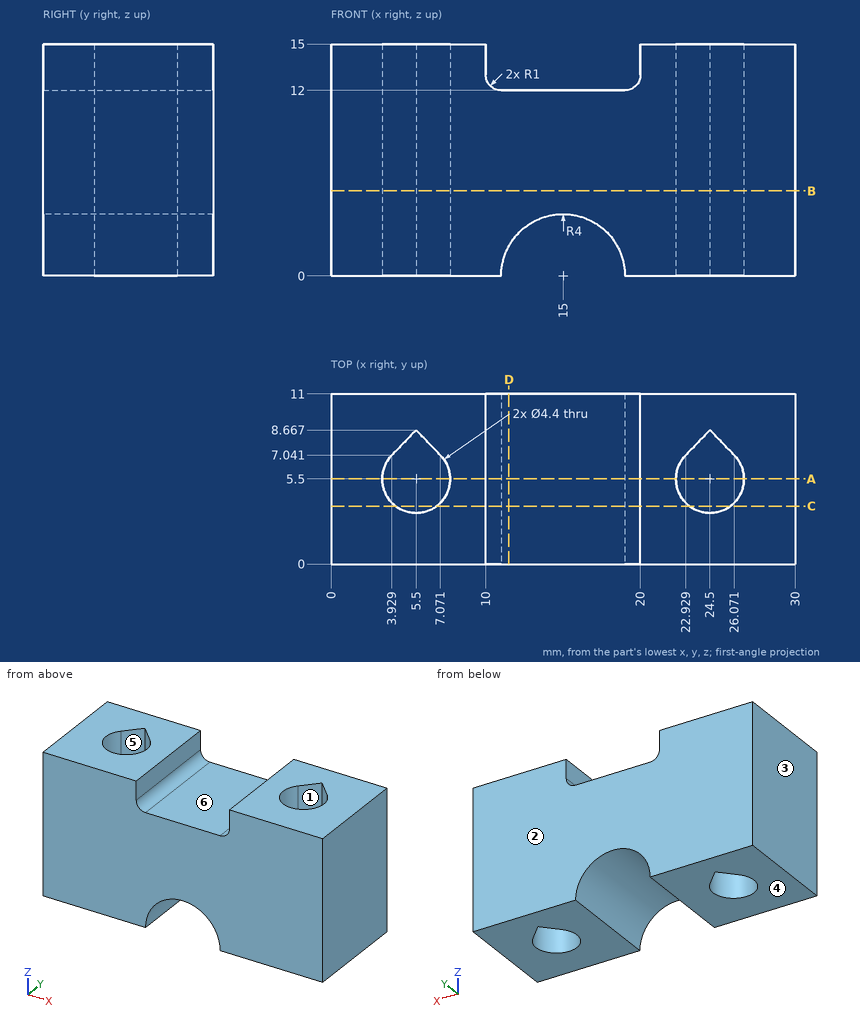
Study the drawing (mm; zero at the part's minimum x, y, z) and answer. A direction names the side the tool comes from. Give positions to 0.01 mm unless a question says otherwise; leave off trailing zeros. Loops run counter-clockwise (first coordinate to the right, second up) from the corner with the lowest first, then second, coordinate; pieces in that order, holes last. Notation, with made-up numbers: M 84.25,-30 L 116.25,-30 A28 ccw 116.25,0 Z; hole C 54,88.25 d9. An arc over 180 degrees is marked long. One line per item, written item: value.
1. Section D-D on x = 11.5 is taken. Determine the outline of the cut face in (y, z), plus the area to 3 significant figures.
Found:
outline: M 0,1.94 L 11,1.94 L 11,12 L 0,12 Z
area: 111 mm^2
2. Find the intervals of material crossed by probe 1 along X at (y, z) = (5.5, 9.25); probe 2 along X at (y, z) = (1.5, 14); probe 3 along X at (y, z) = (6.5, 4.5), in increasing order.
Found:
probe 1: 0 to 3.3, 7.7 to 22.3, 26.7 to 30
probe 2: 0 to 10, 20 to 30
probe 3: 0 to 3.54, 7.46 to 22.54, 26.46 to 30
3. Section A-A on y = 5.5 is taken. Determine the outline of the cut face in (x, z).
Found:
outline: M 0,0 L 3.3,0 L 3.3,15 L 0,15 Z; M 7.7,0 L 11,0 A4 cw 19,0 L 22.3,0 L 22.3,15 L 20,15 L 20,13 A1 cw 19,12 L 11,12 A1 cw 10,13 L 10,15 L 7.7,15 Z; M 26.7,0 L 30,0 L 30,15 L 26.7,15 Z
4. Section C-C on y = 3.75 is taken. Determine the outline of the cut face in (x, z).
Found:
outline: M 0,0 L 4.17,0 L 4.17,15 L 0,15 Z; M 6.83,0 L 11,0 A4 cw 19,0 L 23.17,0 L 23.17,15 L 20,15 L 20,13 A1 cw 19,12 L 11,12 A1 cw 10,13 L 10,15 L 6.83,15 Z; M 25.83,0 L 30,0 L 30,15 L 25.83,15 Z
5. Section B-B on z = 5.5 is taken. Determine the outline of the cut face in (x, y), plus the area to 3 significant figures.
Found:
outline: M 0,0 L 30,0 L 30,11 L 0,11 Z; hole M 3.93,7.04 A2.2 ccw long 7.07,7.04 L 5.5,8.67 Z; hole M 22.93,7.04 A2.2 ccw long 26.07,7.04 L 24.5,8.67 Z
area: 297 mm^2
6. For the marked faces 4, 5 and 6, determine the directions among +Z, -Z, +X, -X, +Y, -Y from which every point of the face is accessible in a straight line to the end or side of a thin tool.
Found:
face 4: -Z, +X, -X, +Y, -Y
face 5: +Z, -Z
face 6: +Z, +Y, -Y
7. For a pull along X with two mould halves and no side action, classify the marked faces 1, 2 and 3 as pulls with the +X half, pulls with the -X half, needs draft (parallel to the pull), parting line crosses it, or undercut.
Found:
face 1: undercut
face 2: needs draft
face 3: pulls with the -X half
8. Each of these flat-tipped pins is pushed along its axis until it touches: P1, Ø2.5, axis at x = 24.5, y = 5.5, coming from the -Z side; P2, Ø2.5, axis at x = 13.5, y = 7.5, coming from the +Z side. Where does it stop, or does it pass through?
Found:
P1: through
P2: z = 12
